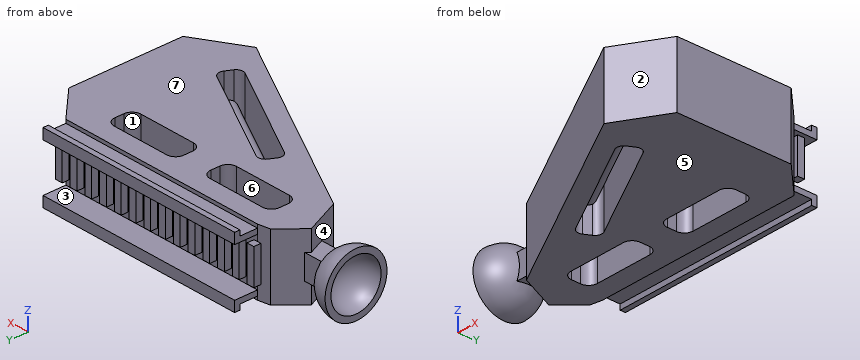
from build123d import *

# Parameters (mm, degrees)
BOSS_EXTRUDE1_DEPTH     = 37
CUT_EXTRUDE1_DEPTH      = 37
CUT_EXTRUDE1_DEPTH_BACK = 1
SKETCH13_W              = 4.25
SKETCH13_H              = 20
BOSS_EXTRUDE3_DEPTH     = 4
REVOLVE4_ANGLE          = 180
BOSS_EXTRUDE5_START     = 1.719088
SKETCH24_W              = 14
SKETCH24_H              = 12
BOSS_EXTRUDE5_DEPTH     = 13.336158
BOSS_EXTRUDE6_DEPTH     = 120
CUT_EXTRUDE2_DEPTH      = 37


with BuildPart() as part:
    # Sketch8 → Boss-Extrude1 (new body)
    with BuildSketch(Plane.XY):
        Polygon((0, 18.749877704), (-119.999774223, 18.749877704), (-126.751399414, 17.492106186), (-138.175152238, 4.606192282), (-128.930068484, -16.486854671), (-8.930236022, -81.486624843), (18.749877704, -64.999999997), (18.749877704, 0), align=None)
    extrude(amount=BOSS_EXTRUDE1_DEPTH)

    # Sketch10 → Cut-Extrude1 (cut, two sides)
    with BuildSketch(Plane.XY) as cut_extrude1_sk:
        with BuildLine():
            Line((-50.945075891, -7.596026142), (-17.985230256, -7.596026142))
            ThreePointArc((-17.985230256, -7.596026142), (-14.44969635, -6.131560048), (-12.985230256, -2.596026142))
            Line((-12.985230256, -2.596026142), (-12.985230256, 2.596026142))
            ThreePointArc((-12.985230256, 2.596026142), (-14.44969635, 6.131560048), (-17.985230256, 7.596026142))
            Line((-17.985230256, 7.596026142), (-50.945075891, 7.596026142))
            ThreePointArc((-50.945075891, 7.596026142), (-54.480609797, 6.131560048), (-55.945075891, 2.596026142))
            Line((-55.945075891, 2.596026142), (-55.945075891, -2.596026142))
            ThreePointArc((-55.945075891, -2.596026142), (-54.480609797, -6.131560048), (-50.945075891, -7.596026142))
        make_face()
        with BuildLine():
            Line((-110.945075891, 7.596026142), (-77.985230256, 7.596026142))
            ThreePointArc((-77.985230256, 7.596026142), (-74.44969635, 6.131560048), (-72.985230256, 2.596026142))
            Line((-72.985230256, 2.596026142), (-72.985230256, -2.596026142))
            ThreePointArc((-72.985230256, -2.596026142), (-74.44969635, -6.131560048), (-77.985230256, -7.596026142))
            Line((-77.985230256, -7.596026142), (-110.945075891, -7.596026142))
            ThreePointArc((-110.945075891, -7.596026142), (-114.480609797, -6.131560048), (-115.945075891, -2.596026142))
            Line((-115.945075891, -2.596026142), (-115.945075891, 2.596026142))
            ThreePointArc((-115.945075891, 2.596026142), (-114.480609797, 6.131560048), (-110.945075891, 7.596026142))
        make_face()
    extrude(amount=CUT_EXTRUDE1_DEPTH, mode=Mode.SUBTRACT)
    extrude(cut_extrude1_sk.sketch, amount=-CUT_EXTRUDE1_DEPTH_BACK, mode=Mode.SUBTRACT)

    # Sketch13 → Boss-Extrude3 (add)
    with BuildSketch(Plane(origin=(0, 18.749877704, 0), x_dir=(1, 0, 0), z_dir=(0, 1, 0))):
        with Locations((0, -18.5)):
            Rectangle(SKETCH13_W, SKETCH13_H)
        with Locations((-9.23, -18.5)):
            Rectangle(SKETCH13_W, SKETCH13_H)
        with Locations((-18.46, -18.5)):
            Rectangle(SKETCH13_W, SKETCH13_H)
        with Locations((-27.69, -18.5)):
            Rectangle(SKETCH13_W, SKETCH13_H)
        with Locations((-36.92, -18.5)):
            Rectangle(SKETCH13_W, SKETCH13_H)
        with Locations((-46.15, -18.5)):
            Rectangle(SKETCH13_W, SKETCH13_H)
        with Locations((-55.38, -18.5)):
            Rectangle(SKETCH13_W, SKETCH13_H)
        with Locations((-64.61, -18.5)):
            Rectangle(SKETCH13_W, SKETCH13_H)
        with Locations((-73.84, -18.5)):
            Rectangle(SKETCH13_W, SKETCH13_H)
        with Locations((-83.07, -18.5)):
            Rectangle(SKETCH13_W, SKETCH13_H)
        with Locations((-92.3, -18.5)):
            Rectangle(SKETCH13_W, SKETCH13_H)
        with Locations((-101.53, -18.5)):
            Rectangle(SKETCH13_W, SKETCH13_H)
        with Locations((-110.76, -18.5)):
            Rectangle(SKETCH13_W, SKETCH13_H)
        with Locations((-119.99, -18.5)):
            Rectangle(SKETCH13_W, SKETCH13_H)
    extrude(amount=BOSS_EXTRUDE3_DEPTH)



with BuildPart() as body_2:
    # Sketch23 → Revolve4 (revolve)
    with BuildSketch(Plane.ZY.offset(162.115)):
        with BuildLine():
            Line((18.502309671, 18.552772626), (18.502309671, 15.181416266))
            ThreePointArc((18.502309671, 15.181416266), (4.238878914, 0.917985509), (18.502309671, -13.345445248))
            Line((18.502309671, -13.345445248), (18.502309671, -16.716801609))
            ThreePointArc((18.502309671, -16.716801609), (0.867522554, 0.917985509), (18.502309671, 18.552772626))
        make_face()
    revolve(axis=Axis((-162.115, 19.719780597, 18.502309671), (0, -1, 0)), revolution_arc=REVOLVE4_ANGLE)


with BuildPart() as part_1:
    add(part.part)

    add(body_2.part)  # Boss-Extrude5 merges body 2
    # Sketch24 → Boss-Extrude5 (add)
    with BuildSketch(Plane.ZY.offset(132.115).offset(BOSS_EXTRUDE5_START)):
        with Locations((18.502309671, 0.701872922)):
            Rectangle(SKETCH24_W, SKETCH24_H)
    extrude(amount=BOSS_EXTRUDE5_DEPTH)

    # Sketch25 → Boss-Extrude6 (add)
    with BuildSketch(Plane(origin=(0, 0, 0), x_dir=(0, 0, -1), z_dir=(1, 0, 0))):
        Polygon((-32, 31.749877704), (-32, 18.749877704), (-35, 18.749877704), (-35, 28.749877704), (-38, 28.749877704), (-38, 31.749877704), align=None)
        Polygon((1, 31.749877704), (-5, 31.749877704), (-5, 18.749877704), (-2, 18.749877704), (-2, 28.749877704), (1, 28.749877704), align=None)
    extrude(amount=-BOSS_EXTRUDE6_DEPTH)

    # Sketch26 → Cut-Extrude2 (cut)
    with BuildSketch(Plane.XY):
        with BuildLine():
            Line((-82.157166646, -21.371866468), (-84.205180797, -25.15282376))
            ThreePointArc((-84.205180797, -25.15282376), (-84.522155627, -28.19783771), (-82.593140666, -30.575122775))
            Line((-82.593140666, -30.575122775), (-22.030526844, -63.379801738))
            ThreePointArc((-22.030526844, -63.379801738), (-18.985512893, -63.696776568), (-16.608227828, -61.767761607))
            Line((-16.608227828, -61.767761607), (-14.560213677, -57.986804316))
            ThreePointArc((-14.560213677, -57.986804316), (-14.243238847, -54.941790365), (-16.172253808, -52.5645053))
            Line((-16.172253808, -52.5645053), (-76.73486763, -19.759826338))
            ThreePointArc((-76.73486763, -19.759826338), (-79.779881581, -19.442851507), (-82.157166646, -21.371866468))
        make_face()
    extrude(amount=CUT_EXTRUDE2_DEPTH, mode=Mode.SUBTRACT)

    # Sketch27 → Revolve-Thin1 (revolve)
    with BuildSketch(Plane.XY.offset(18.5)):
        Polygon((-83.181173721, -23.262345114), (-15.584220753, -59.877282961), (-13.67909131, -56.360113388), (-81.276044279, -19.745175541), align=None)
    revolve(axis=Axis((-83.181173721, -23.262345114, 18.5), (0.879292393, -0.476282361, 0)))


solid = part_1.part
The listing builds one solid part. Answer for the finished solid, in the listing's coordinates (mm). Face numbers are marked on the shaded views. A direction names the side the tool comes from. Give positions to 0.01 mm unless a question says otherwise; leave off trailing zeros. Write each loop counter-clockwise with the first axis right and the second up, starting at its lowest first coordinate (ties: lowest second). Pieces come first, ordered by that corner, then holes.
Item 1: Section C-C, the plane y = -67.5 is taken. Write down the section's boundary in (x, z), plus the area to 3 significant figures.
Item 2: Section A-A, the plane x = -32 is taken. Count the separate pieces of the cut face and the enclosed holes in it, plus the area to 3 significant figures.
Item 3: Find the intervals of material crossed by line 1 along Y through (x, z) = (-23.5, 22); line 2 along Y through (x, z) = (-103, 22.5); line 3 along X through (y, z) = (-51.5, 20.5), in increasing order.
Item 4: Which of the six approach directions +Z, -Z, +X, -X, +Y, -Y give full straight-line access (tool end or side, diameter ignored) to the marked faces 4, 5, 6 and 7?
Item 5: Determine the mould class of the marked faces 1, 2 and 3 for opening direction X: released by +X, released by -X, zero draft, split by the parting line, or undercut.
Item 6: Flat-ended cylindrical pins translate along their axes: P1, Ø8, axis at x = -34.5, y = 23, coming from the -Z side; P2, Ø1.2, axis at y = 21.5, z = 16.5, coming from the -X side (3 decimals); P3, Ø13, axis at x = -137, y = -1, coming from the +Z side. Find the tip coordinate at first contact, or state that the pin passes through.
Completed:
1. outline: (-34.75, 0) - (14.55, 0) - (14.55, 37) - (-34.75, 37) - close
1. area: 1,820 mm2
2. separate pieces: 4
2. enclosed holes: 0
2. area: 2,320 mm2
3. line 1: y = -73.59 to -62.58, -57.79 to -53.39, -48.6 to -7.6, 7.6 to 18.75
3. line 2: y = -30.53 to -7.6, 7.6 to 22.75
3. line 3: x = -64.29 to -43.96, -38.32 to -23.78, -18.14 to 18.75
4. face 4: -Y
4. face 5: -Z, +X, -X, -Y
4. face 6: +Z, -Z
4. face 7: +Z, +X, -X, -Y
5. face 1: undercut
5. face 2: released by +X
5. face 3: zero draft
6. P1: stops at z = 2
6. P2: stops at x = -122.115
6. P3: stops at z = 37
